For this review, take the finished solid that the model builds, in its own axes (mm). Face numbers are marked on the shaded views. A direction names the side the tool comes from. Give positions to 0.01 mm unless a question says otherwise; leave off trailing zeros. Order: outer loops, then holes, each group sorted by start corner. A loop starts at its lowest first (then second) coordinate and runs counter-clockwise, first axis right, second up. Notation, with made-up numbers: (26, 55) - (80, 55) arc R21 cw to (80, 69) - close; hole circle Ø1 at (28, 60.5). An arc over 180 degrees is marked (long way). One line per item, written item: value.
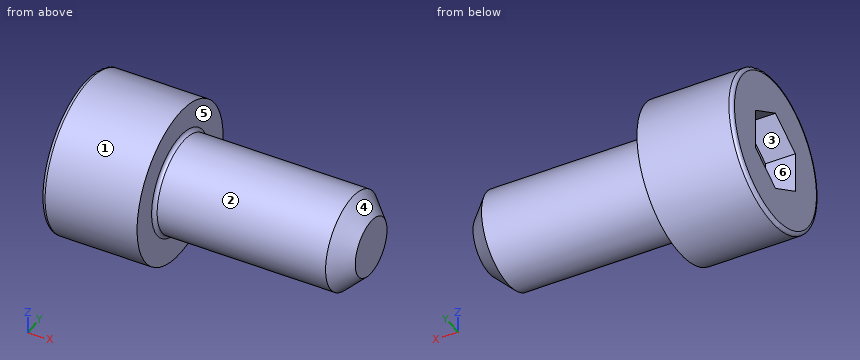
```python
from build123d import *

# Parameters (mm, degrees)
CUT_EXTRUDE_1_DEPTH = 2.5
FILLET_1_R          = 0.3
CHAMFER_1_SIZE      = 1.6


with BuildPart() as part:
    # Эскиз1 → Повернуть1 (revolve)
    with BuildSketch(Plane.XY):
        Polygon((0, 0), (0, 6.5), (8, 6.5), (8, 4), (24, 4), (24, 0), align=None)
    revolve(axis=Axis((24, 0, 0), (-1, 0, 0)))

    # Эскиз2 → Вырез-Вытянуть1 (cut)
    with BuildSketch(Plane.ZY):
        Polygon((-1.732050808, 3), (-3.464101615, 0), (-1.732050808, -3), (1.732050808, -3), (3.464101615, 0), (1.732050808, 3), align=None)
    extrude(amount=-CUT_EXTRUDE_1_DEPTH, mode=Mode.SUBTRACT)

    # Скругление1
    fillet_1_edges = [part.edges().sort_by_distance(p)[0] for p in [
        (8, -4, 0),
        (0, -6.5, 0),
    ]]
    fillet(fillet_1_edges, radius=FILLET_1_R)

    # Фаска1
    chamfer_1_edges = [part.edges().sort_by_distance(p)[0] for p in [
        (24, -4, 0),
    ]]
    chamfer(chamfer_1_edges, length=CHAMFER_1_SIZE)


solid = part.part
```
(1) Machinability: for the marked faces 1, 2 and 3, which of the approach directions +Z, -Z, +X, -X, +Y, -Y give a long, thin tool a straight path to every point of the face, cutting with its end or side? Answer none if there is none.
Answers below:
face 1: +X, -X
face 2: +X
face 3: -X
(2) Take a section at A-A (z = 0). Write out the cut boundary in (x, y), then the cut area to 3 significant figures.
Answers below:
outline: (0, -6.2) arc R0.3 ccw to (0.3, -6.5) - (8, -6.5) - (8, -4.3) arc R0.3 cw to (8.3, -4) - (22.4, -4) - (24, -2.4) - (24, 2.4) - (22.4, 4) - (8.3, 4) arc R0.3 cw to (8, 4.3) - (8, 6.5) - (0.3, 6.5) arc R0.3 ccw to (0, 6.2) - (0, 3) - (2.5, 3) - (2.5, -3) - (0, -3) - close
area: 214 mm^2
(3) Wall thickness on line 1 (X direction, y = 3, z = -4.25); line 2 (X direction, y = -1.75, z = 1.5); line 3 (Z direction, x = 2.75, y = -2.5): over which ranges is each line inside the solid? List them lowest first. Write a range as from..to.
Answers below:
line 1: x = 0..8
line 2: x = 2.5..24
line 3: z = -6..6
(4) For P1, Ø1.2, axis at x = 2, z = 1, coming from the -Y side; P2, Ø1.8, axis at y = -1.5, z = -0.5, coming from the -X side; P3, Ø1.5, axis at x = 17, z = 4, coming from the -Y side, all flat-tipped, find the tip position at first contact; note any pin that passes through.
Answers below:
P1: stops at y = -6.49
P2: stops at x = 2.5
P3: stops at y = -2.33
(5) Draft analysis for pull direction Y (two halves, no side actions). For the marked faces 4, 5 and 6, state which applies: pulls with the +Y half, pulls with the -Y half, needs draft (parallel to the pull), parting line crosses it, or undercut.
Answers below:
face 4: parting line crosses it
face 5: needs draft
face 6: undercut
(6) Take a section at B-B (x = 7). Write out the cut boundary in (y, z), then the cut area to 3 significant figures.
Answers below:
outline: circle Ø13 at (0, 0)
area: 133 mm^2
(7) Take a section at C-C (x = 12.25). Write out the cut boundary in (y, z), then the cut area to 3 significant figures.
Answers below:
outline: circle Ø8 at (0, 0)
area: 50.3 mm^2
